Verification items for the finished model (mm, model axes). Coordinates: 2 decimals unless noted, no trailing zeros. Order: outer loops, then holes, each group sorted by start corner. A loop starts at its lowest first (then second) coordinate and runs counter-clockwise, first axis right, second up. Notation, with made-up numbers: M 9,16.25 L 31,16.25 A33 cw 31,47.25 Z; hole C -16,66.5 d6. An arc over 180 degrees is marked long. Return JSON: item names as keys, results as strings.
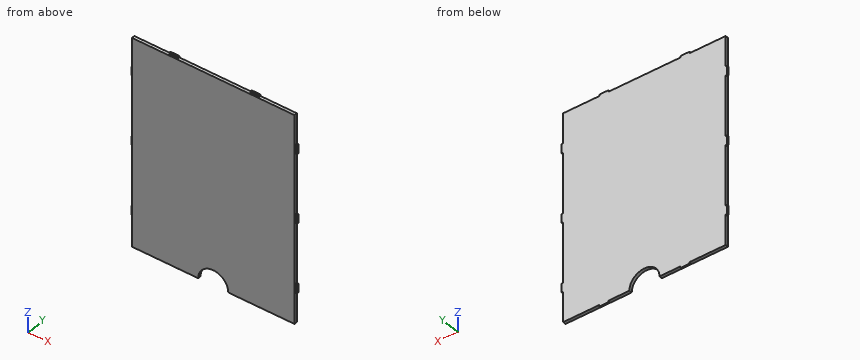
```python
from build123d import *

# Parameters (mm, degrees)
SKETCH1_W           = 54
SKETCH1_H           = 69
BOSS_EXTRUDE1_DEPTH = 1
BOSS_EXTRUDE2_START = -0.5
SKETCH3_W           = 0.5
SKETCH3_H           = 3
BOSS_EXTRUDE2_DEPTH = 0.5
SKETCH4_R           = 5
CUT_EXTRUDE1_DEPTH  = 1


with BuildPart() as part:
    # Sketch1 → Boss-Extrude1 (new body)
    with BuildSketch(Plane.XZ.offset(-34.2740501)):
        with Locations((-40.101257217, 62.307503177)):
            Rectangle(SKETCH1_W, SKETCH1_H)
    extrude(amount=-BOSS_EXTRUDE1_DEPTH)

    # Sketch3 → Boss-Extrude2 (add)
    with BuildSketch(Plane.XZ.offset(-34.2740501).offset(BOSS_EXTRUDE2_START)):
        with Locations((-67.351257217, 85.307503177)):
            Rectangle(SKETCH3_W, SKETCH3_H)
        with Locations((-12.851257217, 85.307503177)):
            Rectangle(SKETCH3_W, SKETCH3_H)
        with Locations((-12.851257217, 62.307503177)):
            Rectangle(SKETCH3_W, SKETCH3_H)
        Polygon((-13.101257217, 39.307503177), (-13.101257217, 37.807503177), (-12.601257217, 37.807503177), (-12.601257217, 40.807503177), (-13.101257217, 40.807503177), align=None)
        Polygon((-25.101261235, 27.80403111), (-26.601257217, 27.807503177), (-28.101261235, 27.807503177), (-28.102410554, 27.310976583), (-25.102418591, 27.304032449), align=None)
        Polygon((-52.101261235, 27.80403111), (-53.601257217, 27.807503177), (-55.101261235, 27.807503177), (-55.102410554, 27.310976583), (-52.102418591, 27.304032449), align=None)
        with Locations((-67.351257217, 39.307503177)):
            Rectangle(SKETCH3_W, SKETCH3_H)
        with Locations((-67.351257217, 62.307503177)):
            Rectangle(SKETCH3_W, SKETCH3_H)
        Polygon((-55.102410554, 97.30402977), (-52.102418591, 97.310973905), (-52.101261235, 96.810975244), (-55.101253198, 96.80403111), align=None)
        Polygon((-28.102410554, 97.30402977), (-25.102418591, 97.310973905), (-25.101261235, 96.810975244), (-28.101253198, 96.80403111), align=None)
    extrude(amount=-BOSS_EXTRUDE2_DEPTH)

    # Sketch4 → Cut-Extrude1 (cut)
    with BuildSketch(Plane.XZ.offset(-34.2740501)):
        with Locations((-40.101257217, 27.807503177)):
            Circle(SKETCH4_R)
    extrude(amount=-CUT_EXTRUDE1_DEPTH, mode=Mode.SUBTRACT)


solid = part.part
```
Q1. Go/stop test with flat-tipped pins: pin 1 (0.6 mm diameter, centred on x = -12.5, y = 35, fed in from -Z); pin 2 (0.5 mm diameter, centred on x = -57.5, y = 35, fed in from -Z). Record where each tip stops, or that it passes through.
Values:
{"pin 1": "z = 37.81", "pin 2": "z = 27.81"}
Q2. Material ranges on line 1 along Z through (x, y) = (-30.5, 34.9); line 2 along X through (y, z) = (35.15, 52); line 3 along X through (y, z) = (34.7, 30.5), recorded low to high.
Values:
{"line 1": "27.81 to 96.81", "line 2": "-67.1 to -13.1", "line 3": "-67.1 to -44.31, -35.89 to -13.1"}
Q3. Cross-section at A-A, the plane z = 72.5. Record the boundary of the cut face in (x, y).
Values:
{"outline": "M -67.1,34.27 L -13.1,34.27 L -13.1,35.27 L -67.1,35.27 Z"}
